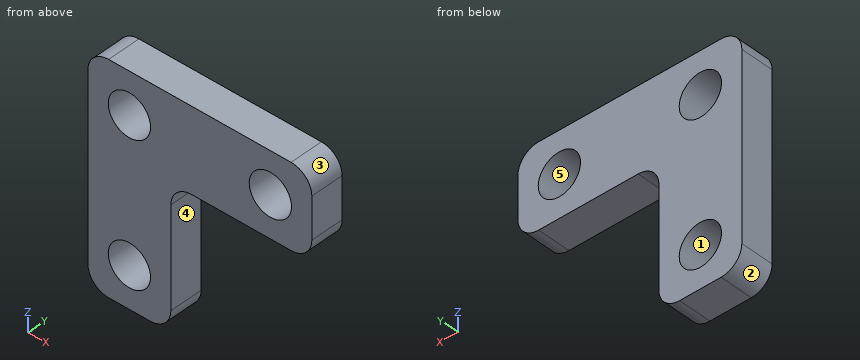
```python
from build123d import *

# Parameters (mm, degrees)
SKETCH1_R           = 2.55
BOSS_EXTRUDE1_DEPTH = 4


with BuildPart() as part:
    # Sketch1 → Boss-Extrude1 (new body)
    with BuildSketch(Plane(origin=(0, 0, 0), x_dir=(1, 0, 0), z_dir=(0, 1, 0))):
        with BuildLine():
            Line((0, 2.5), (0, 24.5))
            ThreePointArc((0, 24.5), (0.732233047, 26.267766953), (2.5, 27))
            Line((2.5, 27), (7.5, 27))
            ThreePointArc((7.5, 27), (9.267766953, 26.267766953), (10, 24.5))
            Line((10, 24.5), (10, 12.5))
            ThreePointArc((10, 12.5), (10.732233047, 10.732233047), (12.5, 10))
            Line((12.5, 10), (24.5, 10))
            ThreePointArc((24.5, 10), (26.267766953, 9.267766953), (27, 7.5))
            Line((27, 7.5), (27, 2.5))
            ThreePointArc((27, 2.5), (26.267766953, 0.732233047), (24.5, 0))
            Line((24.5, 0), (2.5, 0))
            ThreePointArc((2.5, 0), (0.732233047, 0.732233047), (0, 2.5))
        make_face()
        with Locations(Location((22, 5, 0), (0, 0, 270))):
            Circle(SKETCH1_R, mode=Mode.SUBTRACT)
        with Locations(Location((5, 5, 0), (0, 0, 270))):
            Circle(SKETCH1_R, mode=Mode.SUBTRACT)
        with Locations(Location((5, 22, 0), (0, 0, 270))):
            Circle(SKETCH1_R, mode=Mode.SUBTRACT)
    extrude(amount=BOSS_EXTRUDE1_DEPTH)


solid = part.part
```
Model file for the job. Use its own axes, mm. Face numbers are marked on the shaded views. A direction names the side the tool comes from. Give positions to 0.01 mm unless a question says otherwise; leave off trailing zeros. Loops run counter-clockwise (first coordinate to the right, second up) from the corner with the lowest first, then second, coordinate; pieces in that order, holes last. Notation, with made-up numbers: M 39,79.5 L 51,79.5 A18 cw 51,107.5 Z; hole C -13.5,7.5 d3. An arc over 180 degrees is marked long. Use one line per item in the form item = value.
Item 1: Slice it at D-D on y = 1.15. List the corners of the cut face in (x, z).
Filled in:
outline = M 0,-24.5 A2.5 ccw 2.5,-27 L 7.5,-27 A2.5 ccw 10,-24.5 L 10,-12.5 A2.5 cw 12.5,-10 L 24.5,-10 A2.5 ccw 27,-7.5 L 27,-2.5 A2.5 ccw 24.5,0 L 2.5,0 A2.5 ccw 0,-2.5 Z; hole C 5,-22 d5.1; hole C 5,-5 d5.1; hole C 22,-5 d5.1
Item 2: Drill centre lines: L1, parallel to X at y = 3.25, z = -5; L2, parallel to X at y = 1.05, z = -22; L3, parallel to Z at x = 14.5, y = 0.45. Where is each one in solid material? Low to high.
Filled in:
L1 = 0 to 2.45, 7.55 to 19.45, 24.55 to 27
L2 = 0 to 2.45, 7.55 to 10
L3 = -10 to 0
Item 3: Slice it at A-A on x = 5. List the corners of the cut face in (y, z), and give its area (3 significant figures).
Filled in:
outline = M 0,-27 L 4,-27 L 4,-24.55 L 0,-24.55 Z; M 0,-19.45 L 4,-19.45 L 4,-7.55 L 0,-7.55 Z; M 0,-2.45 L 4,-2.45 L 4,0 L 0,0 Z
area = 67.2 mm^2
Item 4: Which spindle directions (+Z, -Z, +X, -X, +Y, -Y) get a long thin tool onto all of the face, cutting with end or side? Do the marked faces 4 and 5. Say none if no direction does.
Filled in:
face_4 = -Z, +X, +Y, -Y
face_5 = +Y, -Y
Item 5: Two-plate mould, pull along X, no slides. Class the marked faces 1, 2 and 3: released by +X, released by -X, zero draft, split by the parting line, or undercut.
Filled in:
face_1 = undercut
face_2 = released by -X
face_3 = released by +X
Item 6: Slice it at C-C on z = -22. List the corners of the cut face in (x, y), and give its area (3 significant figures).
Filled in:
outline = M 0,0 L 2.45,0 L 2.45,4 L 0,4 Z; M 7.55,0 L 10,0 L 10,4 L 7.55,4 Z
area = 19.6 mm^2
Item 7: Slice it at B-B on z = -5. List the corners of the cut face in (x, y).
Filled in:
outline = M 0,0 L 2.45,0 L 2.45,4 L 0,4 Z; M 7.55,0 L 19.45,0 L 19.45,4 L 7.55,4 Z; M 24.55,0 L 27,0 L 27,4 L 24.55,4 Z
Item 8: Flat gauge pin, fed straight in: pin 1 Ø4 at (x, z) = (5, -5) entering from -Y (1 decimal). Where does the tip first touch, or does it go through?
Filled in:
pin_1 = through
